Source: CAD feature listing. Evaluate the final solid. Frame: model axes, mm. Coordinates: 2 decimals unless noted, no trailing zeros. Write each loop counter-clockwise with the first axis right and the second up, starting at its lowest first coordinate (ties: lowest second). Pieces come first, ordered by that corner, then holes. Notation, with made-up numbers: (85.25, -13.75) - (129.25, -13.75) arc R12 ccw to (129.25, 7.25) - close; hole circle Ø8 at (6.5, 18). An arc over 180 degrees is marked (long way). One line per item, written item: value.
from build123d import *

# Parameters (mm, degrees)
SKETCH1_W           = 3.8
SKETCH1_H           = 8
BOSS_EXTRUDE1_DEPTH = 3.45
BOSS_EXTRUDE3_START = -0.5
BOSS_EXTRUDE3_DEPTH = 0.5
CHAMFER2_SIZE       = 0.5
SKETCH8_RX          = 2.494560644
SKETCH8_RY          = 0.718935273
CUT_EXTRUDE2_DEPTH  = 0.05
CUT_EXTRUDE3_DEPTH  = 0.05


# Read off the part's stored shape, not the designer's step: Boss-Extrude3
with BuildPart() as part:
    # Sketch1 → Boss-Extrude1 (new, symmetric)
    with BuildSketch(Plane.XY):
        Rectangle(SKETCH1_W, SKETCH1_H)
    extrude(amount=BOSS_EXTRUDE1_DEPTH, both=True)

    # Boss-Extrude3 outline → Boss-Extrude3 (add)
    with BuildSketch(Plane.XY.offset(3.45).offset(BOSS_EXTRUDE3_START)):
        with BuildLine():
            ThreePointArc((0.386782268, 4.576881383), (0, 4.785801899), (-0.386782268, 4.576881383))
            add(Edge.make_bspline(
                [(-0.386782268, 4.576881383), (-0.522104533, 4.370469494), (-0.576485167, 4.110258291), (-1.543568904, 4.182658763), (-1.9, 4)],
                knots=[0, 0, 0, 0, 0, 1, 1, 1, 1, 1], degree=4))
            Line((-1.9, 4), (1.9, 4))
            add(Edge.make_bspline(
                [(1.9, 4), (1.543568904, 4.182658763), (0.576485167, 4.110258291), (0.522104533, 4.370469494), (0.386782268, 4.576881383)],
                knots=[0, 0, 0, 0, 0, 1, 1, 1, 1, 1], degree=4))
        make_face()
    extrude(amount=BOSS_EXTRUDE3_DEPTH)

    # Chamfer2
    chamfer2_edges = [part.edges().sort_by_distance(p)[0] for p in [
        (0, -4, 3.45),
        (0, -4, -3.45),
        (1.9, -4, 0),
        (-1.9, -4, 0),
    ]]
    chamfer(chamfer2_edges, length=CHAMFER2_SIZE)

    # Sketch8 → Cut-Extrude2 (cut, symmetric)
    with BuildSketch(Plane.XZ.offset(4)):
        with Locations(Location((0, 0), (0, 0, 90))):
            Ellipse(SKETCH8_RX, SKETCH8_RY)
    extrude(amount=CUT_EXTRUDE2_DEPTH, both=True, mode=Mode.SUBTRACT)

    # Sketch9 → Cut-Extrude3 (cut, symmetric)
    with BuildSketch(Plane(origin=(1.9, 0, 0), x_dir=(0, 0, -1), z_dir=(1, 0, 0))):
        Polygon((-1.608695652, 1.52039879), (-1.608695652, 1.67981908), (-1.347826087, 1.67981908), (-1.347826087, 2.32361437), (-1.57495471, 2.20155821), (-1.637681159, 2.3609785), (-1.313405797, 2.52039879), (-1.15942029, 2.52039879), (-1.15942029, 1.67981908), (-0.942028986, 1.67981908), (-0.942028986, 1.52039879), align=None)
        with BuildLine():
            Line((-0.753623188, 1.52039879), (-0.753623188, 1.660117993))
            Line((-0.753623188, 1.660117993), (-0.512681159, 1.893587196))
            add(Edge.make_bspline(
                [(-0.512681159, 1.893587196), (-0.5018156, 1.904159463), (-0.481039355, 1.924374897), (-0.452427524, 1.954418318), (-0.426714142, 1.981714894), (-0.404257947, 2.007005685), (-0.384911278, 2.030762388), (-0.367887318, 2.052940622), (-0.35307316, 2.073689639), (-0.340721742, 2.093374099), (-0.330364569, 2.111983404), (-0.322256202, 2.129907311), (-0.31575837, 2.146967443), (-0.309698908, 2.168941676), (-0.305493732, 2.196715837), (-0.304731855, 2.219056371), (-0.304347826, 2.230317268)],
                knots=[0, 0, 0, 0, 1.561346149, 2.985479849, 4.272660798, 5.42387168, 6.4681479, 7.427594435, 8.303382019, 9.092890023, 9.820107477, 10.495077279, 11.117492523, 11.698467986, 12.839897307, 14, 14, 14, 14], degree=3))
            add(Edge.make_bspline(
                [(-0.304347826, 2.230317268), (-0.304749324, 2.239951277), (-0.305544487, 2.259031359), (-0.312869331, 2.286419819), (-0.32389769, 2.31167432), (-0.340192786, 2.333284373), (-0.360528944, 2.351500926), (-0.381140537, 2.36269725), (-0.399534406, 2.369207499), (-0.414564764, 2.372786302), (-0.430554514, 2.375179437), (-0.44156686, 2.375372066), (-0.447237319, 2.375471254)],
                knots=[0, 0, 0, 0, 1.259052347, 2.493543675, 3.687736162, 4.846054809, 6.008246034, 7.237941048, 7.888132915, 8.5593184, 9.258166694, 10, 10, 10, 10], degree=3))
            add(Edge.make_bspline(
                [(-0.447237319, 2.375471254), (-0.456988906, 2.375134553), (-0.476209579, 2.374470906), (-0.504504735, 2.370167962), (-0.531680703, 2.362610737), (-0.557705297, 2.352017107), (-0.583009083, 2.339296512), (-0.607369703, 2.324204601), (-0.631341549, 2.307520425), (-0.646378777, 2.294899268), (-0.653985507, 2.288514732)],
                knots=[0, 0, 0, 0, 1.020414048, 2.011267059, 2.986668027, 3.96497488, 4.94697347, 5.946696085, 6.961316025, 8, 8, 8, 8], degree=3))
            Line((-0.653985507, 2.288514732), (-0.753623188, 2.408759297))
            add(Edge.make_bspline(
                [(-0.753623188, 2.408759297), (-0.742518604, 2.418001221), (-0.72030534, 2.436488477), (-0.68431817, 2.460977212), (-0.646234813, 2.482437605), (-0.606269993, 2.50111137), (-0.564434736, 2.516559351), (-0.520470754, 2.52692615), (-0.474936737, 2.533905774), (-0.443942977, 2.534559711), (-0.42821558, 2.534891543)],
                knots=[0, 0, 0, 0, 0.971414743, 1.943187718, 2.923163908, 3.90905488, 4.908116413, 5.916732171, 6.942871654, 8, 8, 8, 8], degree=3))
            add(Edge.make_bspline(
                [(-0.42821558, 2.534891543), (-0.416203685, 2.534703898), (-0.392650983, 2.534335966), (-0.358220001, 2.530579803), (-0.325504013, 2.524775686), (-0.294589327, 2.516626165), (-0.265532929, 2.506251119), (-0.2384809, 2.493601472), (-0.213635967, 2.478599538), (-0.191054535, 2.461304731), (-0.17078899, 2.441689013), (-0.15269922, 2.419840212), (-0.137363523, 2.395482265), (-0.124395242, 2.368994948), (-0.113833889, 2.340452893), (-0.106835404, 2.309612456), (-0.102028057, 2.27681502), (-0.101645917, 2.254188651), (-0.101449275, 2.242545529)],
                knots=[0, 0, 0, 0, 1.159472778, 2.273472863, 3.340013536, 4.365414322, 5.356781803, 6.31537468, 7.244130825, 8.153815157, 9.055875647, 9.962049253, 10.886103095, 11.828148954, 12.805810483, 13.817047342, 14.876691883, 16, 16, 16, 16], degree=3))
            add(Edge.make_bspline(
                [(-0.101449275, 2.242545529), (-0.101573271, 2.232797158), (-0.10181811, 2.213548196), (-0.105266832, 2.185201632), (-0.109988074, 2.157717091), (-0.117468921, 2.131299919), (-0.126556111, 2.105586764), (-0.13745779, 2.08027856), (-0.150492092, 2.055452632), (-0.164982926, 2.030681159), (-0.181295483, 2.006109055), (-0.19988108, 1.981983737), (-0.219700719, 1.957357861), (-0.241779881, 1.933018624), (-0.265556322, 1.908393081), (-0.290302007, 1.882559449), (-0.317355297, 1.856767431), (-0.335891122, 1.839304984), (-0.345335145, 1.830407848)],
                knots=[0, 0, 0, 0, 0.945736526, 1.867434716, 2.768631143, 3.650402628, 4.528787893, 5.414963327, 6.32280855, 7.249039709, 8.200182995, 9.183579422, 10.204429958, 11.268168642, 12.372135405, 13.527717836, 14.740369513, 16, 16, 16, 16], degree=3))
            Line((-0.345335145, 1.830407848), (-0.492753623, 1.694311833))
            Line((-0.492753623, 1.694311833), (-0.072463768, 1.694311833))
            Line((-0.072463768, 1.694311833), (-0.072463768, 1.52039879))
            Line((-0.072463768, 1.52039879), (-0.753623188, 1.52039879))
        make_face()
        Polygon((1.400362319, 1.52039879), (1.151268116, 1.52039879), (0.847826087, 2.52039879), (1.061141304, 2.52039879), (1.228713768, 1.918270167), (1.282608696, 1.720806399), (1.338088768, 1.92959263), (1.502717391, 2.52039879), (1.702898551, 2.52039879), align=None)
    extrude(amount=CUT_EXTRUDE3_DEPTH, both=True, mode=Mode.SUBTRACT)


solid = part.part
1) Section query A-A on z = 2.75. Output: boundary loops of the cut face in (x, y).
Values found:
outline: (-1.9, -3.5) - (-1.4, -4) - (1.4, -4) - (1.9, -3.5) - (1.9, 4) - (-1.9, 4) - close
2) Draft query along Z for faces 1 (the flat face through (0, 4, 0)), 2 (the flat face through (0, 1, 3.45)), 3 (the flat face through (0, -3.95, 0)). Return one class per face: released by +Z, released by -Z, zero draft, split by the parting line, or undercut.
Values found:
face 1: zero draft
face 2: released by +Z
face 3: undercut
3) Material intervals for line 1 (Y direction, x = -0.35, z = 1); line 2 (Z direction, x = 0.2, y = 4.25); line 3 (Y direction, x = -1.7, z = -1), sorted ascending.
Values found:
line 1: -3.95 to 4
line 2: 2.95 to 3.45
line 3: -3.7 to 4
4) Contact query for a flat-ended pin moving along its axis: P1, Ø0.7, axis at x = 0, z = 1, coming from the -Y side. Output: stop coordinate, or through.
Values found:
P1: y = -3.95
